Design review of the part built by this model. Coordinates are the model's own, in mm. A direction names the side the tool comes from. Coordinates: 2 decimals unless noted, no trailing zeros. Loops run counter-clockwise (first coordinate to the right, second up) from the corner with the lowest first, then second, coordinate; pieces in that order, holes last. Notation, with made-up numbers: M 46,-11 L 101,-11 A14 cw 101,15 Z; hole C 42,57.25 d3. An arc over 180 degrees is marked long. One line per item, written item: value.
```python
from build123d import *

# Parameters (mm, degrees)
F0_W     = 200
F0_H     = 150
F1_DEPTH = 2
F2_W     = 148
F2_H     = 2
F2_W_2   = 25.5013404053
F3_DEPTH = 300
F5_DEPTH = 2.001
F6_R     = 3.85
F7_DEPTH = 2


with BuildPart() as f1:
    # F0 (on Top) → F1 (new body)
    with BuildSketch(Plane.XY):
        with Locations((0.4986595947, -11.6955466568)):
            Rectangle(F0_W, F0_H)
    extrude(amount=F1_DEPTH)

    # F2 (on face) → F3 (join)
    with BuildSketch(Plane.XY.offset(2)):
        with Locations((0, -11.6955466568)):
            Rectangle(F2_W, F2_H)
        Polygon((100.4986595947, -10.6955466568), (74, -10.6955466568), (74, -12.6955466568), (100.4986595947, -12.6955466568), (100.4986595947, -11.6955466568), align=None)
        with Locations((-86.7506702027, -11.6955466568)):
            Rectangle(F2_W_2, F2_H)
    extrude(amount=F3_DEPTH)

    # F2 (on face) → F5 (cut, through all)
    with BuildSketch(Plane.XY.offset(2)):
        with BuildLine():
            Line((-71, -31.6955466568), (-74, -31.6955466568))
            Line((-74, -31.6955466568), (-74, -34.6955466568))
            ThreePointArc((-74, -34.6955466568), (-71.8786796564, -33.8168670004), (-71, -31.6955466568))
        make_face()
        with BuildLine():
            ThreePointArc((-71, -31.6955466568), (-71.8786796564, -29.5742263133), (-74, -28.6955466568))
            Line((-74, -28.6955466568), (-74, -31.6955466568))
            Line((-74, -31.6955466568), (-71, -31.6955466568))
        make_face()
        with BuildLine():
            ThreePointArc((-74, -28.6955466568), (-76.1213203436, -29.5742263133), (-77, -31.6955466568))
            Line((-77, -31.6955466568), (-74, -31.6955466568))
            Line((-74, -31.6955466568), (-74, -28.6955466568))
        make_face()
        with BuildLine():
            Line((-74, -31.6955466568), (-77, -31.6955466568))
            ThreePointArc((-77, -31.6955466568), (-76.1213203436, -33.8168670004), (-74, -34.6955466568))
            Line((-74, -34.6955466568), (-74, -31.6955466568))
        make_face()
        with BuildLine():
            Line((74, -31.6955466568), (74, -28.6955466568))
            ThreePointArc((74, -28.6955466568), (71.8786796564, -29.5742263133), (71, -31.6955466568))
            Line((71, -31.6955466568), (74, -31.6955466568))
        make_face()
        with BuildLine():
            Line((74, -31.6955466568), (71, -31.6955466568))
            ThreePointArc((71, -31.6955466568), (71.8786796564, -33.8168670004), (74, -34.6955466568))
            Line((74, -34.6955466568), (74, -31.6955466568))
        make_face()
        with BuildLine():
            Line((77, -31.6955466568), (74, -31.6955466568))
            Line((74, -31.6955466568), (74, -34.6955466568))
            ThreePointArc((74, -34.6955466568), (76.1213203436, -33.8168670004), (77, -31.6955466568))
        make_face()
        with BuildLine():
            ThreePointArc((77, -31.6955466568), (76.1213203436, -29.5742263133), (74, -28.6955466568))
            Line((74, -28.6955466568), (74, -31.6955466568))
            Line((74, -31.6955466568), (77, -31.6955466568))
        make_face()
        with BuildLine():
            ThreePointArc((-71, 8.3044533432), (-71.8786796564, 10.4257736867), (-74, 11.3044533432))
            Line((-74, 11.3044533432), (-74, 8.3044533432))
            Line((-74, 8.3044533432), (-71, 8.3044533432))
        make_face()
        with BuildLine():
            Line((-71, 8.3044533432), (-74, 8.3044533432))
            Line((-74, 8.3044533432), (-74, 5.3044533432))
            ThreePointArc((-74, 5.3044533432), (-71.8786796564, 6.1831329996), (-71, 8.3044533432))
        make_face()
        with BuildLine():
            Line((-74, 8.3044533432), (-77, 8.3044533432))
            ThreePointArc((-77, 8.3044533432), (-76.1213203436, 6.1831329996), (-74, 5.3044533432))
            Line((-74, 5.3044533432), (-74, 8.3044533432))
        make_face()
        with BuildLine():
            ThreePointArc((-74, 11.3044533432), (-76.1213203436, 10.4257736867), (-77, 8.3044533432))
            Line((-77, 8.3044533432), (-74, 8.3044533432))
            Line((-74, 8.3044533432), (-74, 11.3044533432))
        make_face()
        with BuildLine():
            Line((77, 8.3044533432), (74, 8.3044533432))
            Line((74, 8.3044533432), (74, 5.3044533432))
            ThreePointArc((74, 5.3044533432), (76.1213203436, 6.1831329996), (77, 8.3044533432))
        make_face()
        with BuildLine():
            ThreePointArc((77, 8.3044533432), (76.1213203436, 10.4257736867), (74, 11.3044533432))
            Line((74, 11.3044533432), (74, 8.3044533432))
            Line((74, 8.3044533432), (77, 8.3044533432))
        make_face()
        with BuildLine():
            Line((74, 8.3044533432), (74, 11.3044533432))
            ThreePointArc((74, 11.3044533432), (71.8786796564, 10.4257736867), (71, 8.3044533432))
            Line((71, 8.3044533432), (74, 8.3044533432))
        make_face()
        with BuildLine():
            Line((74, 5.3044533432), (74, 8.3044533432))
            Line((74, 8.3044533432), (71, 8.3044533432))
            ThreePointArc((71, 8.3044533432), (71.8786796564, 6.1831329996), (74, 5.3044533432))
        make_face()
    extrude(amount=-F5_DEPTH, mode=Mode.SUBTRACT)

    # F6 (on face) → F7 (cut)
    with BuildSketch(Plane(origin=(0, -10.6955466568, 0), x_dir=(-1, 0, 0), z_dir=(0, 1, 0))):
        with Locations((-41.8486595947, 102)):
            Circle(F6_R)
        with Locations((36.9513404053, 102)):
            Circle(F6_R)
    extrude(amount=-F7_DEPTH, mode=Mode.SUBTRACT)


solid = f1.part
```
(1) We need section D-D on z = 45. State the section outline as (x, y) points, then the cut area to 3 significant figures.
Reply:
outline: M -99.5,-12.7 L 100.5,-12.7 L 100.5,-10.7 L -99.5,-10.7 Z
area: 400 mm2
(2) To check wall thickness, follow line 1 along Z through (x, y) = (-46.5, 28); line 2 along Y through (x, z) = (11, 139). State the ranges of each line that lie inside material, in increasing order. Write a range as [from, to].
Reply:
line 1: z = [0, 2]
line 2: y = [-12.7, -10.7]
(3) We need section B-B on x = 27. State the section outline as (y, z) points, then the cut area to 3 significant figures.
Reply:
outline: M -86.7,0 L 63.3,0 L 63.3,2 L -10.7,2 L -10.7,302 L -12.7,302 L -12.7,2 L -86.7,2 Z
area: 900 mm2
(4) Insertion check: pin 1 (12.5 mm diameter, centred on x = -36.95, z = 102, fed in from +Y); pin 2 (22 mm diameter, centred on x = 38.5, y = 16, fed in from +Z); pin 3 (10 mm diameter, centred on x = 41.85, z = 102, fed in from -Y). Each pin has a flat end and moves straight along its axis. Give the tip position at first contact, or say it passes through.
Reply:
pin 1: stops at y = -10.7
pin 2: stops at z = 2
pin 3: stops at y = -12.7
(5) Mouldability with a two-part tool opening along X and no side actions: class faces 4 (the cylindrical face through (-40.51, -11.68, 100.53)), 5 (the flat face through (-99.501, -12, 150)), 6 (the flat face through (-1, -12.696, 150)) as released by +X, released by -X, zero draft, split by the parting line, or undercut.
Reply:
face 4: undercut
face 5: released by -X
face 6: zero draft
(6) Tool access review of faces 1 (the flat face through (-1, -11, 0)), 2 (the flat face through (2, -10.696, 150)), 3 (the flat face through (-1, -49, 2)): name each direction out of +Z, -Z, +X, -X, +Y, -Y from which nothing blocks a thin tool from reaching the whole face with its end or side.
Reply:
face 1: -Z, +X, -X, +Y, -Y
face 2: +Z, +X, -X, +Y
face 3: +Z, +X, -X, -Y
(7) We need section C-C on y = 44. State the section outline as (x, z) points, then the cut area to 3 significant figures.
Reply:
outline: M -99.5,0 L 100.5,0 L 100.5,2 L -99.5,2 Z
area: 400 mm2
(8) We need section A-A on z = 102. State the section outline as (x, y) points, then the cut area to 3 significant figures.
Reply:
outline: M -99.5,-12.7 L -40.8,-12.7 L -40.8,-10.7 L -99.5,-10.7 Z; M -33.1,-12.7 L 38,-12.7 L 38,-10.7 L -33.1,-10.7 Z; M 45.7,-12.7 L 100.5,-12.7 L 100.5,-10.7 L 45.7,-10.7 Z
area: 369 mm2
